Read the model definition and answer for the solid it produces. Units are mm, in the model's axes. A direction names the side the tool comes from. Give positions to 0.01 mm unless a question says otherwise; leave off trailing zeros. Loops run counter-clockwise (first coordinate to the right, second up) from the corner with the lowest first, then second, coordinate; pieces in that order, holes last. Notation, with made-up numbers: (65, 62.5) -> (91, 62.5) arc R34 cw to (91, 94.5) -> close; hole circle Ø3 at (40.25, 27.5). An arc over 180 degrees is marked (long way). One line per item, written item: value. Start each with the question number.
from build123d import *

# Parameters (mm, degrees)
SKETCH1_W           = 70
SKETCH1_H           = 40
BOSS_EXTRUDE1_DEPTH = 21
SKETCH2_R           = 2
BOSS_EXTRUDE2_DEPTH = 10
SKETCH3_R           = 2
BOSS_EXTRUDE3_DEPTH = 10
SKETCH4_R           = 0.85
BOSS_EXTRUDE4_DEPTH = 10


with BuildPart() as part:
    # Sketch1 → Boss-Extrude1 (new body)
    with BuildSketch(Plane(origin=(0, 0, 0), x_dir=(0, 1, 0), z_dir=(0, 0, 1))):
        Rectangle(SKETCH1_W, SKETCH1_H)
    extrude(amount=BOSS_EXTRUDE1_DEPTH)

    # Sketch2 → Boss-Extrude2 (add)
    with BuildSketch(Plane.XZ.offset(35)):
        with Locations((-6, 16)):
            Circle(SKETCH2_R)
        with Locations((0, 16)):
            Circle(SKETCH2_R)
        with Locations((6, 16)):
            Circle(SKETCH2_R)
    extrude(amount=BOSS_EXTRUDE2_DEPTH)

    # Sketch3 → Boss-Extrude3 (add)
    with BuildSketch(Plane(origin=(0, 35, 0), x_dir=(-1, 0, 0), z_dir=(0, 1, 0))):
        with Locations(Location((-4, 2, 0), (0, 0, 270))):
            Circle(SKETCH3_R)
        with Locations(Location((4, 2, 0), (0, 0, 270))):
            Circle(SKETCH3_R)
    extrude(amount=BOSS_EXTRUDE3_DEPTH)

    # Sketch4 → Boss-Extrude4 (add)
    with BuildSketch(Plane.XY.offset(21)):
        with Locations((18, -27)):
            Circle(SKETCH4_R)
        with Locations((18, -25)):
            Circle(SKETCH4_R)
        with Locations((18, -23)):
            Circle(SKETCH4_R)
        with Locations((18, -21)):
            Circle(SKETCH4_R)
        with Locations((18, -19)):
            Circle(SKETCH4_R)
        with Locations((18, -17)):
            Circle(SKETCH4_R)
        with Locations((18, -5)):
            Circle(SKETCH4_R)
        with Locations((18, -3)):
            Circle(SKETCH4_R)
        with Locations((18, -1)):
            Circle(SKETCH4_R)
        with Locations((18, 1)):
            Circle(SKETCH4_R)
    extrude(amount=BOSS_EXTRUDE4_DEPTH)


solid = part.part
Item 1: Determine the mould class of faces 4 (the flat face through (0, -45, 16)), 5 (the cylindrical face through (17.82, -17.83, 25.93)), 6 (the cylindrical face through (6, -40, 18)) for opening direction Y: pulls with the +Y half, pulls with the -Y half, needs draft (parallel to the pull), parting line crosses it, or undercut.
Item 2: Consider L1, parallel to X at y = -40, z = 15; L2, parallel to Y at x = 16, z = 16.5; L3, parallel to Z at x = -5, y = -22. Determine where each line is inside the solid, lowest interval first. Write a range as [from, to].
Item 3: Flat-ended cylindrical pins translate along their axes: pin 1 (2 mm diameter, centred on x = -14, y = -15, fed in from +Z); pin 2 (8 mm diameter, centred on x = 10.5, z = 20, fed in from +Y); pin 3 (10.5 mm diameter, centred on x = -7, z = 6.5, fed in from -Y). Find the tip coordinate at first contact, or state that the pin passes through.
Item 4: Section A-A, the plane z = 26 is taken. State how many separate pieces and enclosed holes the cut face has, plus the area to 3 significant figures.
Item 5: For faces 1 (the cylindrical face through (5.774, 39.93, 1.077)), 2 (the flat face through (18, -5, 31)), 3 (the cylindrical face through (18.392, -5.754, 25.93)), determine the directions among +Z, -Z, +X, -X, +Y, -Y from which every point of the face is accessible in a straight line to the end or side of a thin tool.
Item 6: Section B-B, the plane x = 0 is taken. Determine the outline of the cut face in (y, z), plus the area to 3 significant figures.
Item 7: Section C-C, the plane y = 1 is taken. Determine the outline of the cut face in (x, z).
Item 8: Section D-D, the plane z = 16 is taken. Determine the outline of the cut face in (x, y).
Computed values:
1. face 4: pulls with the -Y half
1. face 5: undercut
1. face 6: needs draft
2. L1: [-7.73, -4.27], [-1.73, 1.73], [4.27, 7.73]
2. L2: [-35, 35]
2. L3: [0, 21]
3. pin 1: z = 21
3. pin 2: y = 35
3. pin 3: y = -35
4. separate pieces: 10
4. enclosed holes: 0
4. area: 22.7 mm²
5. face 1: +Y
5. face 2: +Z, +X, -X, +Y, -Y
5. face 3: +Z
6. outline: (-45, 14) -> (-35, 14) -> (-35, 0) -> (35, 0) -> (35, 21) -> (-35, 21) -> (-35, 18) -> (-45, 18) -> close
6. area: 1,510 mm²
7. outline: (-20, 0) -> (20, 0) -> (20, 21) -> (18.85, 21) -> (18.85, 31) -> (17.15, 31) -> (17.15, 21) -> (-20, 21) -> close
8. outline: (-20, -35) -> (-8, -35) -> (-8, -45) -> (-4, -45) -> (-4, -35) -> (-2, -35) -> (-2, -45) -> (2, -45) -> (2, -35) -> (4, -35) -> (4, -45) -> (8, -45) -> (8, -35) -> (20, -35) -> (20, 35) -> (-20, 35) -> close
